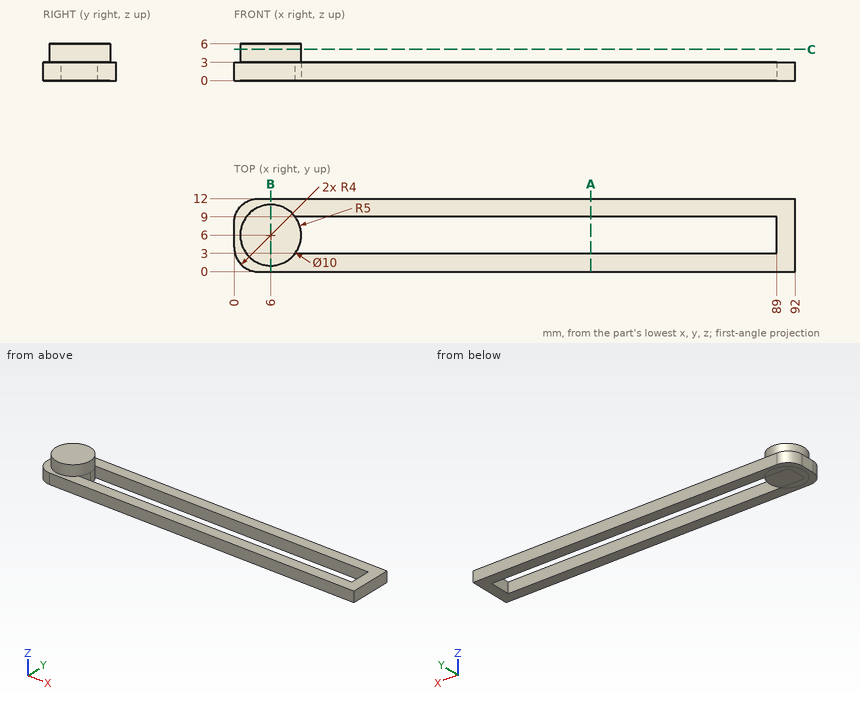
The figure shows three views and two pictorial views of one solid part (mm, origin at its lowest corner). Answer the questions. Round coordinates to 2 decimals unless told otherwise and drop trailing zeros. Order: outer loops, then holes, each group sorted by start corner. A loop starts at its lowest first (then second) coordinate and runs counter-clockwise, first axis right, second up. Notation, with made-up numbers: M 64.5,39 L 98.5,39 A15 cw 98.5,46 Z; hole C 51.25,36.25 d11. An arc over 180 degrees is marked long. Answer in a Markdown table with one row per item. Add a question column.
1) The part is cut by section C-C on z = 5.1. Determine the outline of the cut face in (x, y), plus the area to 3 significant figures.
2) The part is cut by section A-A on x = 58.5. Determine the outline of the cut face in (y, z), plus the area to 3 significant figures.
3) The part is cut by section B-B on x = 6. Determine the outline of the cut face in (y, z), plus the area to 3 significant figures.
4) Consider line 1 along X through (y, z) = (6.25, 1.15); line 2 along Y through (x, z) = (10.5, 2.1); line 3 along Z through (x, y) = (75, 0.5). Determine where each line is inside the solid, lowest interval first. Write a range as from..to.
5) A flat-ended cylindrical pin translates along its axis: pin 1 Ø3 at (y, z) = (6.5, 3.5) entering from +X. Find the tip coordinate at first contact, or state that the pin passes through.
Findings below:
| question | item | result |
|---|---|---|
| 1 | outline | C 6,6 d10 |
| 1 | area | 78.5 mm² |
| 2 | outline | M 0,0 L 3,0 L 3,3 L 0,3 Z; M 9,0 L 12,0 L 12,3 L 9,3 Z |
| 2 | area | 18.0 mm² |
| 3 | outline | M 0,0 L 12,0 L 12,3 L 11,3 L 11,6 L 1,6 L 1,3 L 0,3 Z |
| 3 | area | 66.0 mm² |
| 4 | line 1 | x = 0..10.99, 89..92 |
| 4 | line 2 | y = 0..3, 3.82..8.18, 9..12 |
| 4 | line 3 | z = 0..3 |
| 5 | pin 1 | stops at x = 92 |
